The listing builds one solid part. Answer for the finished solid, in the listing's coordinates (mm). Face numbers are marked on the shaded views. Give positions to 0.01 mm unless a question says otherwise; leave off trailing zeros. Write each loop counter-clockwise with the first axis right and the second up, starting at its lowest first coordinate (ties: lowest second). Pieces come first, ordered by that corner, then holes. Notation, with made-up numbers: (20.25, 70) - (72.25, 70) arc R24 cw to (72.25, 103) - close; hole circle Ø9 at (33, -28). An arc over 180 degrees is marked (long way). One line per question, with ' | ' between items. Start each with the question number.
1. A cutting plane is placed at B-B (y = -33). State how many separate pieces and enclosed holes the cut face has, then the cut area to 3 significant figures.
2. A cutting plane is placed at A-A (z = -3.75). Determine the outline of the cut face in (x, y), then the cut area to 3 significant figures.
3. Find the intervals of material crossed by L1, parallel to Y at x = 0, z = -0.35; L2, parallel to Y at x = 10, z = 0.4; L3, parallel to X at y = -31, z = -0.75, in increasing order. Write a range as from..to.
4. The mould has two halves that part along X. Classify the marked faces 1 and 2: +X half, -X half, draft (parallel to the pull), parting line (faces both ways), or undercut.
5. Given P1, Ø1, axis at x = -31, z = 0, coming from the -Y side; P2, Ø3.5, axis at x = -10, y = 0, coming from the +Z side; P3, Ø13, axis at x = 0, y = 0, coming from the -Z side; P4, Ø1.5, axis at y = 31.5, z = -6, coming from the +X side, each flat-ended and moving along its own axis, determine where each tip first touches the part or whether it passes through.
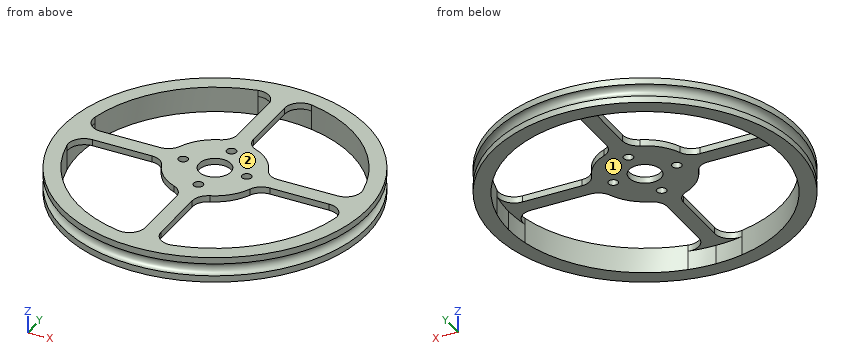
```python
from build123d import *

# Parameters (mm, degrees)
F0_R          = 48
F1_DEPTH      = 1
F1_DEPTH_BACK = 7
F0_R_2        = 1.5
F0_R_3        = 5
F2_DEPTH      = 1
F3_DEPTH      = 1


with BuildPart() as f1:
    # F0 (on Top) → F1 (new body, two sides)
    with BuildSketch(Plane.XY) as f1_sk:
        Circle(F0_R)
        with BuildLine():
            ThreePointArc((8.4868421053, -42.1541636269), (4.2644439289, -42.7880183927), (0, -43))
            ThreePointArc((0, -43), (-4.2644439289, -42.7880183927), (-8.4868421053, -42.1541636269))
            ThreePointArc((-8.4868421053, -42.1541636269), (-30.405591591, -30.405591591), (-42.1541636269, -8.4868421053))
            ThreePointArc((-42.1541636269, -8.4868421053), (-43, 0), (-42.1541636269, 8.4868421053))
            ThreePointArc((-42.1541636269, 8.4868421053), (-30.405591591, 30.405591591), (-8.4868421053, 42.1541636269))
            ThreePointArc((-8.4868421053, 42.1541636269), (0, 43), (8.4868421053, 42.1541636269))
            ThreePointArc((8.4868421053, 42.1541636269), (30.405591591, 30.405591591), (42.1541636269, 8.4868421053))
            ThreePointArc((42.1541636269, 8.4868421053), (42.7880183927, 4.2644439289), (43, 0))
            ThreePointArc((43, 0), (42.7880183927, -4.2644439289), (42.1541636269, -8.4868421053))
            ThreePointArc((42.1541636269, -8.4868421053), (30.405591591, -30.405591591), (8.4868421053, -42.1541636269))
        make_face(mode=Mode.SUBTRACT)
    extrude(amount=F1_DEPTH)
    extrude(f1_sk.sketch, amount=-F1_DEPTH_BACK)



with BuildPart() as f2:
    # F0 (on Top) → F2 (new body, symmetric)
    with BuildSketch(Plane.XY):
        with BuildLine():
            ThreePointArc((0, -15), (2.8652589369, -14.7238001625), (5.625, -13.9053721633))
            ThreePointArc((5.625, -13.9053721633), (10.6066017178, -10.6066017178), (13.9053721633, -5.625))
            ThreePointArc((13.9053721633, -5.625), (14.7238001625, -2.8652589369), (15, 0))
            ThreePointArc((15, 0), (14.7238001625, 2.8652589369), (13.9053721633, 5.625))
            ThreePointArc((13.9053721633, 5.625), (10.6066017178, 10.6066017178), (5.625, 13.9053721633))
            ThreePointArc((5.625, 13.9053721633), (0, 15), (-5.625, 13.9053721633))
            ThreePointArc((-5.625, 13.9053721633), (-10.6066017178, 10.6066017178), (-13.9053721633, 5.625))
            ThreePointArc((-13.9053721633, 5.625), (-15, 0), (-13.9053721633, -5.625))
            ThreePointArc((-13.9053721633, -5.625), (-10.6066017178, -10.6066017178), (-5.625, -13.9053721633))
            ThreePointArc((-5.625, -13.9053721633), (-2.8652589369, -14.7238001625), (0, -15))
        make_face()
        with Locations((0, -10)):
            Circle(F0_R_2, mode=Mode.SUBTRACT)
        with Locations((-10, 0)):
            Circle(F0_R_2, mode=Mode.SUBTRACT)
        Circle(F0_R_3, mode=Mode.SUBTRACT)
        with Locations((10, 0)):
            Circle(F0_R_2, mode=Mode.SUBTRACT)
        with Locations((0, 10)):
            Circle(F0_R_2, mode=Mode.SUBTRACT)
    extrude(amount=F2_DEPTH, both=True)


with BuildPart() as f1_1:
    add(f1.part)

    add(f2.part)  # F3 merges F2
    # F0 (on Top) → F3 (join, symmetric)
    with BuildSketch(Plane.XY):
        with BuildLine():
            Line((0, -43), (0, -15))
            ThreePointArc((0, -15), (-2.8652589369, -14.7238001625), (-5.625, -13.9053721633))
            ThreePointArc((-5.625, -13.9053721633), (-3.3542190121, -15.7454112459), (-2.5, -18.5404962177))
            Line((-2.5, -18.5404962177), (-2.5, -37.2525166935))
            ThreePointArc((-2.5, -37.2525166935), (-4.3325254955, -41.1212510167), (-8.4868421053, -42.1541636269))
            ThreePointArc((-8.4868421053, -42.1541636269), (-4.2644439289, -42.7880183927), (0, -43))
        make_face()
        with BuildLine():
            ThreePointArc((2.5, -18.5404962177), (3.3542190121, -15.7454112459), (5.625, -13.9053721633))
            ThreePointArc((5.625, -13.9053721633), (2.8652589369, -14.7238001625), (0, -15))
            Line((0, -15), (0, -43))
            ThreePointArc((0, -43), (4.2644439289, -42.7880183927), (8.4868421053, -42.1541636269))
            ThreePointArc((8.4868421053, -42.1541636269), (4.3325254955, -41.1212510167), (2.5, -37.2525166935))
            Line((2.5, -37.2525166935), (2.5, -18.5404962177))
        make_face()
        with BuildLine():
            ThreePointArc((15, 0), (14.7238001625, -2.8652589369), (13.9053721633, -5.625))
            ThreePointArc((13.9053721633, -5.625), (15.7454112459, -3.3542190121), (18.5404962177, -2.5))
            Line((18.5404962177, -2.5), (37.2525166935, -2.5))
            ThreePointArc((37.2525166935, -2.5), (41.1212510167, -4.3325254955), (42.1541636269, -8.4868421053))
            ThreePointArc((42.1541636269, -8.4868421053), (42.7880183927, -4.2644439289), (43, 0))
            Line((43, 0), (15, 0))
        make_face()
        with BuildLine():
            ThreePointArc((13.9053721633, 5.625), (14.7238001625, 2.8652589369), (15, 0))
            Line((15, 0), (43, 0))
            ThreePointArc((43, 0), (42.7880183927, 4.2644439289), (42.1541636269, 8.4868421053))
            ThreePointArc((42.1541636269, 8.4868421053), (41.1212510167, 4.3325254955), (37.2525166935, 2.5))
            Line((37.2525166935, 2.5), (18.5404962177, 2.5))
            ThreePointArc((18.5404962177, 2.5), (15.7454112459, 3.3542190121), (13.9053721633, 5.625))
        make_face()
        with BuildLine():
            ThreePointArc((-5.625, 13.9053721633), (0, 15), (5.625, 13.9053721633))
            ThreePointArc((5.625, 13.9053721633), (3.3542190121, 15.7454112459), (2.5, 18.5404962177))
            Line((2.5, 18.5404962177), (2.5, 37.2525166935))
            ThreePointArc((2.5, 37.2525166935), (4.3325254955, 41.1212510167), (8.4868421053, 42.1541636269))
            ThreePointArc((8.4868421053, 42.1541636269), (0, 43), (-8.4868421053, 42.1541636269))
            ThreePointArc((-8.4868421053, 42.1541636269), (-4.3325254955, 41.1212510167), (-2.5, 37.2525166935))
            Line((-2.5, 37.2525166935), (-2.5, 18.5404962177))
            ThreePointArc((-2.5, 18.5404962177), (-3.3542190121, 15.7454112459), (-5.625, 13.9053721633))
        make_face()
        with BuildLine():
            ThreePointArc((-18.5404962177, -2.5), (-15.7454112459, -3.3542190121), (-13.9053721633, -5.625))
            ThreePointArc((-13.9053721633, -5.625), (-15, 0), (-13.9053721633, 5.625))
            ThreePointArc((-13.9053721633, 5.625), (-15.7454112459, 3.3542190121), (-18.5404962177, 2.5))
            Line((-18.5404962177, 2.5), (-37.2525166935, 2.5))
            ThreePointArc((-37.2525166935, 2.5), (-41.1212510167, 4.3325254955), (-42.1541636269, 8.4868421053))
            ThreePointArc((-42.1541636269, 8.4868421053), (-43, 0), (-42.1541636269, -8.4868421053))
            ThreePointArc((-42.1541636269, -8.4868421053), (-41.1212510167, -4.3325254955), (-37.2525166935, -2.5))
            Line((-37.2525166935, -2.5), (-18.5404962177, -2.5))
        make_face()
    extrude(amount=F3_DEPTH, both=True)

    # F4 (on Right) → F5 (revolve, cut)
    with BuildSketch(Plane.YZ):
        with BuildLine():
            Line((48, -4.95), (48, -1.05))
            ThreePointArc((48, -1.05), (46.05, -3), (48, -4.95))
        make_face()
    revolve(axis=Axis((0, 0, -3.6724961751), (0, 0, -1)), mode=Mode.SUBTRACT)


solid = f1_1.part
```
Determined:
1) separate pieces: 3 | enclosed holes: 0 | area: 110 mm2
2) outline: circle Ø92.4 at (0, 0); hole circle Ø86 at (0, 0) | area: 897 mm2
3) L1: -48..-11.5, -8.5..-5, 5..8.5, 11.5..48 | L2: -46.95..-41.82, -11.18..-1.5, 1.5..11.18, 41.82..46.95 | L3: -36.65..-29.8, -2.5..2.5, 29.8..36.65
4) face 1: undercut | face 2: draft
5) P1: y = -37.06 | P2: z = 1 | P3: z = -1 | P4: x = 36.86
